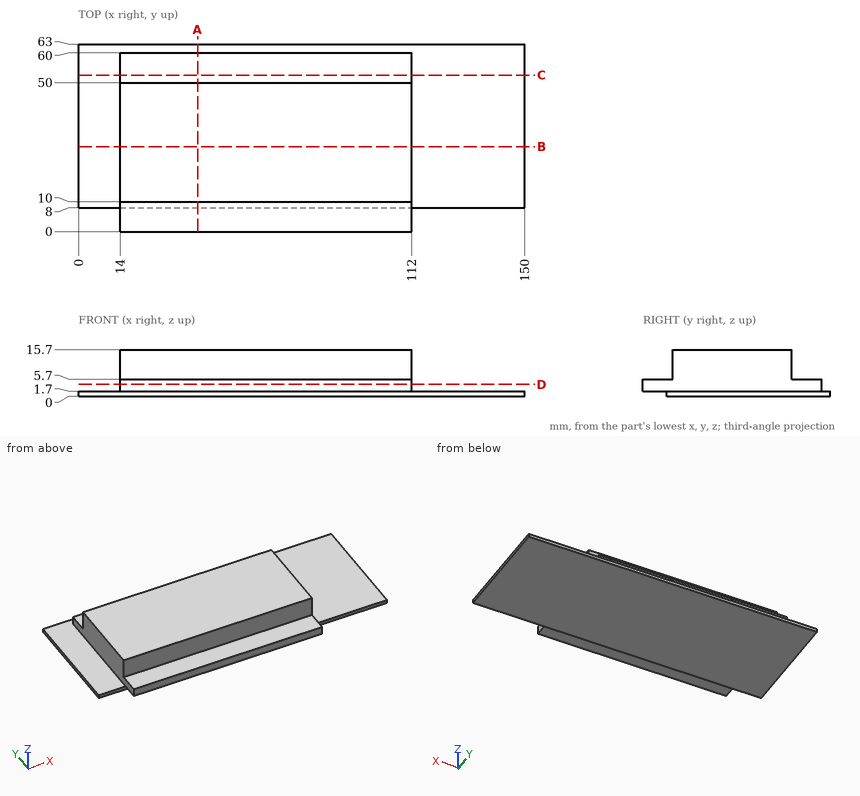
Part print with two shaded views. Sizes in mm from the minimum x, y, z corner. Round coordinates to 2 decimals unless told otherwise and drop trailing zeros. Order: outer loops, then holes, each group sorted by start corner. A loop starts at its lowest first (then second) coordinate and runs counter-clockwise, first axis right, second up.
(1) Band-saw the part on A-A (x = 40). List the corners of the cut face in (y, z), then the cut area to 4 significant figures.
(2) Band-saw the part on B-B (y = 28.5). List the corners of the cut face in (x, z).
(3) Pin check, flat tips, straight feed: pin 1 (2 mm diameter, centred on y = 12, z = 3, fed in from +X); pin 2 (11 mm diameter, centred on x = 65.5, y = 54, fed in from +Z); pin 3 (8 mm diameter, centred on x = 84.5, y = 5, fed in from +Z); pin 4 (4.5 mm diameter, centred on x = 47.5, z = 4, fed in from +Y). Stop position of each tip, or through.
(4) Band-saw the part on C-C (y = 52.5). List the corners of the cut face in (x, z).
(5) Band-saw the part on D-D (z = 4). List the corners of the cut face in (x, y), then the cut area to 3 significant figures.
(6) Drill centre lines: line 1 (X direction, y = 13, z = 15.25); line 2 (Y direction, x = 61, z = 10.75); line 3 (Z direction, x = 130.5, y = 54). Where is each one in solid material? Low to high.
Verdict:
1. outline: (0, 1.7) - (8, 1.7) - (8, 0) - (63, 0) - (63, 1.7) - (60, 1.7) - (60, 5.7) - (50, 5.7) - (50, 15.7) - (10, 15.7) - (10, 5.7) - (0, 5.7) - close
1. area: 733.5 mm2
2. outline: (0, 0) - (150, 0) - (150, 1.7) - (112, 1.7) - (112, 15.7) - (14, 15.7) - (14, 1.7) - (0, 1.7) - close
3. pin 1: stops at x = 112
3. pin 2: stops at z = 15.7
3. pin 3: stops at z = 5.7
3. pin 4: stops at y = 60
4. outline: (0, 0) - (150, 0) - (150, 1.7) - (112, 1.7) - (112, 5.7) - (14, 5.7) - (14, 1.7) - (0, 1.7) - close
5. outline: (14, 0) - (112, 0) - (112, 60) - (14, 60) - close
5. area: 5,880 mm2
6. line 1: x = 14 to 112
6. line 2: y = 10 to 50
6. line 3: z = 0 to 1.7
